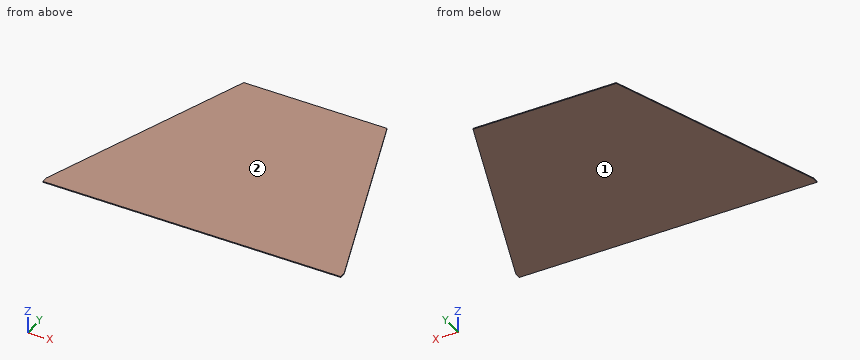
```python
from build123d import *

# Parameters (mm, degrees)
SALIENTE_EXTRUIR1_DEPTH = 1.9
CROQUIS2_W              = 5
CROQUIS2_H              = 30.827719102
CROQUIS2_H_2            = 21.572663196
CORTAR_EXTRUIR1_DEPTH   = 10


with BuildPart() as part:
    # Croquis1 → Saliente-Extruir1 (new body)
    with BuildSketch(Plane.XY):
        Polygon((0, 0), (650, 0), (478.989928337, 469.846310393), (171.010071663, 469.846310393), align=None)
    extrude(amount=SALIENTE_EXTRUIR1_DEPTH)

    # Croquis2 → Cortar-Extruir1 (cut)
    with BuildSketch(Plane.XY.offset(1.9)):
        with Locations((647.5, 15.413859551)):
            Rectangle(CROQUIS2_W, CROQUIS2_H)
        with Locations((2.5, 10.786331598)):
            Rectangle(CROQUIS2_W, CROQUIS2_H_2)
    extrude(amount=-CORTAR_EXTRUIR1_DEPTH, mode=Mode.SUBTRACT)


solid = part.part
```
Here's how the part is built. I have some questions about the finished solid (model axes, mm). Face numbers are marked on the shaded views. Coordinates: 2 decimals unless noted, no trailing zeros. Write each loop counter-clockwise with the first axis right and the second up, starting at its lowest first coordinate (ties: lowest second). Pieces come first, ordered by that corner, then holes. Notation, with made-up numbers: M 49,75.5 L 60,75.5 A19 cw 60,95.5 Z; hole C 8.5,70.5 d3. An arc over 180 degrees is marked long. Answer as CSV lines item,"result". Start each with the question number.
Q1. If we mould it in two halves opening along Z, with no side actions, what happens to the marked faces 1 and 2? For each: pulls with the +Z half, pulls with the -Z half, needs draft (parallel to the pull), parting line crosses it, or undercut.
Q2. Suppose I cut it at A-A, the plane z = 0.4. List the corners of the cut face in (x, y) for me.
Q3. I need wall thicknesses on probe 1 along X at (y, z) = (292, 1.65); probe 2 along X at (y, z) = (204, 0.35). Which ranges of each line are inside material? Lowest first, please. Write a range as [from, to].
Q4. Suppose I cut it at B-B, the plane x = 111. List the corners of the cut face in (y, z) for me.
Q5. Suppose I cut it at C-C, the plane y = 248.5. List the corners of the cut face in (x, z) for me.
Entries:
1,face 1,"pulls with the -Z half"
1,face 2,"pulls with the +Z half"
2,outline,"M 5,0 L 645,0 L 645,13.74 L 478.99,469.85 L 171.01,469.85 L 5,13.74 Z"
3,probe 1,"x = [106.28, 543.72]"
3,probe 2,"x = [74.25, 575.75]"
4,outline,"M 0,0 L 304.97,0 L 304.97,1.9 L 0,1.9 Z"
5,outline,"M 90.45,0 L 559.55,0 L 559.55,1.9 L 90.45,1.9 Z"
